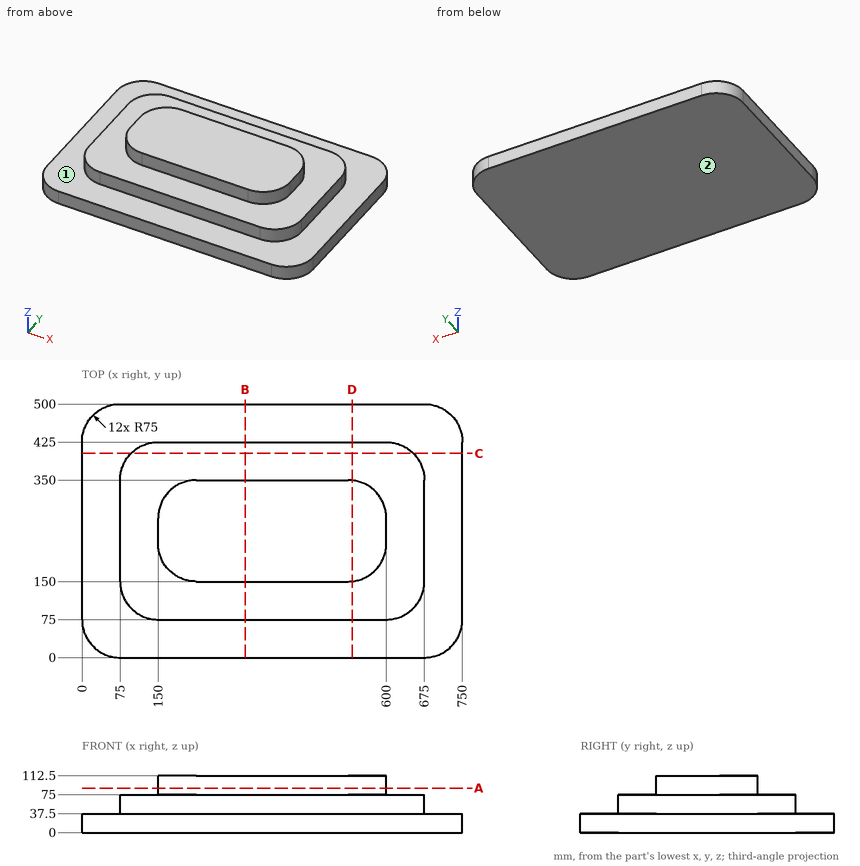
Verification items for this drawing (mm, ordinates from the low corner). A direction names the side the tool comes from. Coordinates: 2 decimals unless noted, no trailing zeros. Loops run counter-clockwise (first coordinate to the right, second up) from the corner with the lowest first, then second, coordinate; pieces in that order, holes last.
Item 1: Sectioned sample at D-D, the plane x = 532.5. Record the boundary of the cut face in (y, z).
Item 2: Thickness scan on line 1 (X direction, y = 195, z = 65); line 2 (Y direction, x = 380, z = 77); line 3 (Z direction, x = 687, y = 416). Record the ranges inside material, lowest first.
Item 3: Go/stop test with flat-tipped pins: pin 1 Ø3 at (y, z) = (160, 65.5) entering from -X; pin 2 Ø19 at (y, z) = (240, 93.5) entering from +X; pin 3 Ø19 at (y, z) = (249, 91) entering from -X. Record where each tip stops, or that it passes through.
Item 4: Sectioned sample at C-C, the plane y = 402.5. Record the boundary of the cut face in (x, z), then the cut area to 3 significant figures.
Item 5: Sectioned sample at A-A, the plane z = 88. Record the boundary of the cut face in (x, y).
Item 6: Access from +Z, -Z, +X, -X, +Y, -Y to the whole of each face (thin tool, end or side, straight path). Record for the marked faces 1 and 2.
Item 7: Sectioned sample at B-B, the plane x = 321.5. Record the boundary of the cut face in (y, z).
Check result:
1. outline: (0, 0) - (500, 0) - (500, 37.5) - (425, 37.5) - (425, 75) - (349.62, 75) - (349.62, 112.5) - (150.38, 112.5) - (150.38, 75) - (75, 75) - (75, 37.5) - (0, 37.5) - close
2. line 1: x = 75 to 675
2. line 2: y = 150 to 350
2. line 3: z = 0 to 37.5
3. pin 1: stops at x = 75
3. pin 2: stops at x = 600
3. pin 3: stops at x = 150
4. outline: (0, 0) - (750, 0) - (750, 37.5) - (653.56, 37.5) - (653.56, 75) - (96.44, 75) - (96.44, 37.5) - (0, 37.5) - close
4. area: 49,000 mm2
5. outline: (150, 225) arc R75 ccw to (225, 150) - (525, 150) arc R75 ccw to (600, 225) - (600, 275) arc R75 ccw to (525, 350) - (225, 350) arc R75 ccw to (150, 275) - close
6. face 1: +Z
6. face 2: -Z, +X, -X, +Y, -Y
7. outline: (0, 0) - (500, 0) - (500, 37.5) - (425, 37.5) - (425, 75) - (350, 75) - (350, 112.5) - (150, 112.5) - (150, 75) - (75, 75) - (75, 37.5) - (0, 37.5) - close
